The figure shows three views and two pictorial views of one solid part (mm, origin at its lowest corner). Answer the questions. Coordinates: 2 decimals unless noted, no trailing zeros. Write each loop counter-clockwise with the first axis right and the second up, starting at its lowest first coordinate (ties: lowest second). Pieces come first, ordered by that corner, then holes. Notation, with made-up numbers: M 11,71.25 L 21,71.25 A12 ccw 21,89.25 Z; hole C 12.5,77.25 d6. An arc over 180 degrees is marked long. Use a Markdown table: item, result. Add a question column.
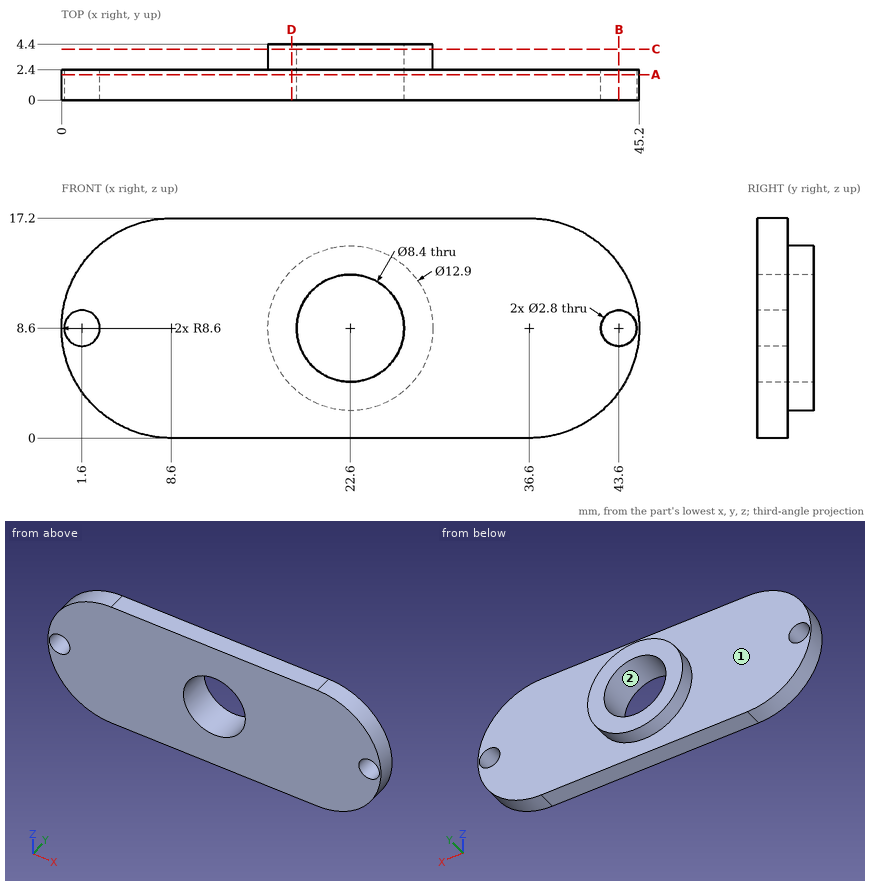
Item 1: Find section B-B on x = 43.6. Give the vertices of the cut face in (y, z).
Item 2: Determine the mould class of the marked faces 1 and 2 for opening direction X: pulls with the +X half, pulls with the -X half, needs draft (parallel to the pull), parting line crosses it, or undercut.
Item 3: Find section A-A on y = 2. Give the vertices of the cut face in (x, z).
Item 4: Consider probe 1 along Z at (x, y) = (22.6, 2.15); probe 2 along X at (y, z) = (3.35, 8.6); probe 3 along X at (y, z) = (1.45, 8.5). Determine where each line is inside the solid, lowest interval first.
Item 5: Each of these flat-tipped pins is pushed along its axis until it touches: pin 1 (6 mm diameter, centred on x = 6.5, z = 10.5, fed in from +Y); pin 2 (2 mm diameter, centred on y = 3, z = 3, fed in from +X); pin 3 (2 mm diameter, centred on x = 43.6, z = 8.6, fed in from -Y). Where does it stop, or does it pass through?
Item 6: Find section C-C on y = 4. Give the vertices of the cut face in (x, z).
Item 7: Find section D-D on x = 18. Give the vertices of the cut face in (y, z).
Geometry says:
| question | item | result |
|---|---|---|
| 1 | outline | M 0,3.6 L 2.4,3.6 L 2.4,7.2 L 0,7.2 Z; M 0,10 L 2.4,10 L 2.4,13.6 L 0,13.6 Z |
| 2 | face 1 | needs draft |
| 2 | face 2 | undercut |
| 3 | outline | M 8.6,0 L 36.6,0 A8.6 ccw 36.6,17.2 L 8.6,17.2 A8.6 ccw Z; hole C 1.6,8.6 d2.8; hole C 22.6,8.6 d8.4; hole C 43.6,8.6 d2.8 |
| 4 | probe 1 | z = 0 to 4.4, 12.8 to 17.2 |
| 4 | probe 2 | x = 16.15 to 18.4, 26.8 to 29.05 |
| 4 | probe 3 | x = 0 to 0.2, 3 to 18.4, 26.8 to 42.2, 45 to 45.2 |
| 5 | pin 1 | stops at y = 2.4 |
| 5 | pin 2 | stops at x = 43.74 |
| 5 | pin 3 | passes through |
| 6 | outline | C 22.6,8.6 d12.9; hole C 22.6,8.6 d8.4 |
| 7 | outline | M 0,0 L 2.4,0 L 2.4,4.08 L 4.4,4.08 L 4.4,13.12 L 2.4,13.12 L 2.4,17.2 L 0,17.2 Z |
